from build123d import *

# Parameters (mm, degrees)
SKETCH1_R              = 4.05
BOSS_EXTRUDE1_DEPTH    = 8
SKETCH2_R              = 10
BOSS_EXTRUDE2_DEPTH    = 10
FILLET1_R              = 1
SKETCH3_R              = 2.55
CUT_EXTRUDE1_DEPTH     = 10
CUT_EXTRUDE2_REACH     = 24.891
M2_5_CLEARANCE_HOLE1_D = 2.9
SKETCH28_R             = 3.5
CUT_EXTRUDE3_DEPTH     = 6.5
SKETCH29_W             = 8.1
SKETCH29_H             = 0.5
CUT_EXTRUDE7_DEPTH     = 23.891046451
FILLET2_R              = 0.25
BOSS_EXTRUDE3_START    = 5
BOSS_EXTRUDE3_DEPTH    = 5
CHAMFER1_SIZE          = 0.5
CUT_EXTRUDE8_DEPTH     = 7
BOSS_EXTRUDE4_START    = -2
BOSS_EXTRUDE4_DEPTH    = 3
CHAMFER2_SIZE          = 0.5
SKETCH35_R             = 4.05
CUT_EXTRUDE9_DEPTH     = 8


with BuildPart() as part:
    # Sketch1 → Boss-Extrude1 (new body)
    with BuildSketch(Plane(origin=(0, 0, 0), x_dir=(1, 0, 0), z_dir=(0, 1, 0))):
        with Locations(Location((0, 0, 0), (0, 0, 270))):
            Circle(SKETCH1_R)
    extrude(amount=BOSS_EXTRUDE1_DEPTH)

    # Sketch2 → Boss-Extrude2 (add)
    with BuildSketch(Plane(origin=(0, 8, 0), x_dir=(1, 0, 0), z_dir=(0, 1, 0))):
        with Locations(Location((0, 0, 0), (0, 0, 270))):
            Circle(SKETCH2_R)
    extrude(amount=BOSS_EXTRUDE2_DEPTH)

    # Fillet1
    fillet1_edges = [part.edges().sort_by_distance(p)[0] for p in [
        (0, 0, -4.05),
        (0, 8, -10),
        (0, 18, -10),
    ]]
    fillet(fillet1_edges, radius=FILLET1_R)

    # Sketch3 → Cut-Extrude1 (cut)
    with BuildSketch(Plane(origin=(0, 18, 0), x_dir=(1, 0, 0), z_dir=(0, 1, 0))):
        with Locations(Location((0, 0, 0), (0, 0, 270))):
            Circle(SKETCH3_R)
    extrude(amount=-CUT_EXTRUDE1_DEPTH, mode=Mode.SUBTRACT)

    # Cut-Extrude2: up to this face of the body (flat: up to its plane)
    cut_extrude2_end = Plane(part.part.faces().sort_by_distance((0, 8, -8.745441559))[0])
    # Sketch20 → Cut-Extrude2 (cut, up to the picked face)
    with BuildSketch(Plane(origin=(0, 18, 0), x_dir=(1, 0, 0), z_dir=(0, 1, 0)), mode=Mode.PRIVATE) as cut_extrude2_sk1:
        with BuildLine():
            Line((-0.75, 2.437211521), (0.75, 2.437211521))
            Line((0.75, 2.437211521), (0.75, 9.971835338))
            ThreePointArc((0.75, 9.971835338), (0, 10), (-0.75, 9.971835338))
            Line((-0.75, 9.971835338), (-0.75, 2.437211521))
        make_face()
    cut_extrude2_tool1 = split(extrude(cut_extrude2_sk1.sketch, amount=-CUT_EXTRUDE2_REACH, mode=Mode.PRIVATE), bisect_by=cut_extrude2_end, keep=Keep.BOTH, mode=Mode.PRIVATE)
    add(cut_extrude2_tool1.solids().sort_by(Axis((0, 18, -6.213919), (0, -1, 0)))[0], mode=Mode.SUBTRACT)

    # M2.5 Clearance Hole1 (through all)
    with Locations(Plane(origin=(10, 0, 0), x_dir=(0, 0, -1), z_dir=(1, 0, 0))):
        with Locations((6.204523429, 13)):
            Hole(M2_5_CLEARANCE_HOLE1_D / 2)

    # Sketch28 → Cut-Extrude3 (cut)
    with BuildSketch(Plane(origin=(10, 0, 0), x_dir=(0, 0, -1), z_dir=(1, 0, 0))):
        with Locations((6.204523429, 13)):
            Circle(SKETCH28_R)
    extrude(amount=-CUT_EXTRUDE3_DEPTH, mode=Mode.SUBTRACT)

    # Sketch29 → Cut-Extrude7 (cut, through all)
    with BuildSketch(Plane.XY):
        with Locations((0, 7.75)):
            Rectangle(SKETCH29_W, SKETCH29_H)
    extrude(amount=-CUT_EXTRUDE7_DEPTH, mode=Mode.SUBTRACT)

    # Fillet2
    fillet2_edges = [part.edges().sort_by_distance(p)[0] for p in [
        (-3.3, 8, 0),
        (3.3, 8, 0),
        (0, 7.5, 0),
    ]]
    fillet(fillet2_edges, radius=FILLET2_R - 0.0001)  # a hair under: the kernel refuses the full size

    # Sketch30 → Boss-Extrude3 (add)
    with BuildSketch(Plane(origin=(0, 18, 0), x_dir=(1, 0, 0), z_dir=(0, 1, 0)).offset(BOSS_EXTRUDE3_START)):
        with BuildLine():
            Line((-0.75, 3.31624788), (-0.75, 2.437211521))
            ThreePointArc((-0.75, 2.437211521), (0, -2.55), (0.75, 2.437211521))
            Line((0.75, 2.437211521), (0.75, 3.31624788))
            ThreePointArc((0.75, 3.31624788), (0, -3.4), (-0.75, 3.31624788))
        make_face()
    extrude(amount=-BOSS_EXTRUDE3_DEPTH)

    # Chamfer1
    chamfer1_edges = [part.edges().sort_by_distance(p)[0] for p in [
        (0, 23, 3.4),
    ]]
    chamfer(chamfer1_edges, length=CHAMFER1_SIZE)

    # Sketch33 → Cut-Extrude8 (cut)
    with BuildSketch(Plane.ZY.offset(10)):
        Polygon((-3.144567003, 13), (-4.674545216, 15.65), (-7.734501643, 15.65), (-9.264479856, 13), (-7.734501643, 10.35), (-4.674545216, 10.35), align=None)
    extrude(amount=-CUT_EXTRUDE8_DEPTH, mode=Mode.SUBTRACT)

    # Sketch34 → Boss-Extrude4 (add)
    with BuildSketch(Plane(origin=(0, 23, 0), x_dir=(1, 0, 0), z_dir=(0, 1, 0)).offset(BOSS_EXTRUDE4_START)):
        with BuildLine():
            Line((-0.75, 3.31624788), (-0.75, 4.132493194))
            ThreePointArc((-0.75, 4.132493194), (0, -4.2), (0.75, 4.132493194))
            Line((0.75, 4.132493194), (0.75, 3.31624788))
            ThreePointArc((0.75, 3.31624788), (0, -3.4), (-0.75, 3.31624788))
        make_face()
    extrude(amount=-BOSS_EXTRUDE4_DEPTH)

    # Chamfer2
    chamfer2_edges = [part.edges().sort_by_distance(p)[0] for p in [
        (0, 21, 4.2),
    ]]
    chamfer(chamfer2_edges, length=CHAMFER2_SIZE)

    # Sketch35 → Cut-Extrude9 (cut)
    with BuildSketch(Plane.XZ):
        Circle(SKETCH35_R)
    extrude(amount=-CUT_EXTRUDE9_DEPTH, mode=Mode.SUBTRACT)


solid = part.part
Here's how the part is built. I have some questions about the finished solid (model axes, mm). A direction names the side the tool comes from. Give positions to 0.01 mm unless a question says otherwise; leave off trailing zeros. Order: outer loops, then holes, each group sorted by start corner. A loop starts at its lowest first (then second) coordinate and runs counter-clockwise, first axis right, second up. Notation, with made-up numbers: (34, -1.75) -> (52, -1.75) arc R28 cw to (52, 32.25) -> close; hole circle Ø10 at (80.5, 4.5). An arc over 180 degrees is marked (long way). Use a Markdown table: item, result. Add a question column.
Item 1: Will these pins go through, and if not, where does the flat tip stop? pin 1 (2 mm diameter, centred on y = 13, z = -5.5, fed in from +X); pin 2 (6 mm diameter, centred on y = 12, z = -5.5, fed in from +X); pin 3 (3 mm diameter, centred on x = 6, y = 13, fed in from +Z).
Item 2: Imagine slicing it at B-B on y = 12.5. Please give me the cut outline in (x, z), plus the area to 3 significant figures.
Item 3: Imagine slicing it at C-C on x = 1.25. Give the number of separate pieces and of enclosed holes in the cut face, plus the area to 3 significant figures.
Item 4: If we mould it in two halves opening along Z, with no side actions, what happens to faces 6 (the face through (-2, 8, 2)), 7 (the face through (0.1, 21.8, 3.4)), 8 (the face through (-3, 14.2, -4.9))? For each: pulls with the +Z half, pulls with the -Z half, needs draft (parallel to the pull), parting line crosses it, or undercut.
Item 5: I need wall thicknesses on line 1 (X direction, y = 11, z = 0); line 2 (X direction, y = 19.45, z = 0); line 3 (Y direction, x = 3, z = -4). Which ranges of each line are inside material? Lowest first, please.
Item 6: Imagine slicing it at D-D on y = 19.5. Please give me the cut outline in (x, z), plus the area to 3 significant figures.
Item 7: For faces 1 (the face through (-6.29, 14.31, -3.9)), 2 (the face through (-1.891, 12.118, -7.355)), 3 (the face through (0.75, 13.9, -4.6)), 4 (the face through (3.5, 15, -6)), 5 (the face through (-2, 18, 4)), which set-ups out of +Z, -Z, +X, -X, +Y, -Y let a thin tool reach every point of the face, with its end or its side?
Item 8: Imagine slicing it at A-A on z = 0. Please give me the cut outline in (x, y), plus the area to 3 significant figures.
Data:
| question | item | result |
|---|---|---|
| 1 | pin 1 | stops at x = 3.5 |
| 1 | pin 2 | stops at x = 9.68 |
| 1 | pin 3 | stops at z = 8.93 |
| 2 | outline | (-9.39, -3.43) -> (-3, -3.43) -> (-3, -4.84) -> (-0.75, -4.84) -> (-0.75, -2.44) arc R2.55 cw (long way) to (0.75, -2.44) -> (0.75, -4.84) -> (3.5, -4.84) -> (3.5, -2.74) -> (9.62, -2.74) arc R10 ccw (long way) to start; (-4.41, -8.98) arc R10 ccw to (-0.75, -9.97) -> (-0.75, -7.57) -> (-3, -7.57) -> (-3, -8.98) -> close; (0.75, -9.97) arc R10 ccw to (3.5, -9.37) -> (3.5, -7.57) -> (0.75, -7.57) -> close |
| 2 | area | 217 mm² |
| 3 | separate pieces | 2 |
| 3 | enclosed holes | 1 |
| 3 | area | 160 mm² |
| 4 | face 6 | needs draft |
| 4 | face 7 | parting line crosses it |
| 4 | face 8 | undercut |
| 5 | line 1 | x = -10 to -2.55, 2.55 to 10 |
| 5 | line 2 | x = -4.2 to -2.55, 2.55 to 4.2 |
| 5 | line 3 | y = 8 to 18 |
| 6 | outline | (-0.75, -4.13) -> (-0.75, -2.44) arc R2.55 cw (long way) to (0.75, -2.44) -> (0.75, -4.13) arc R4.2 ccw (long way) to start |
| 6 | area | 32.5 mm² |
| 7 | face 1 | -X |
| 7 | face 2 | +X, -X |
| 7 | face 3 | -Z, +Y, -Y |
| 7 | face 4 | +X |
| 7 | face 5 | +Y |
| 8 | outline | (-10, 9) arc R1 ccw to (-9, 8) -> (-2.55, 8) -> (-2.55, 23) -> (-2.9, 23) -> (-3.4, 22.5) -> (-3.4, 21) -> (-3.7, 21) -> (-4.2, 20.5) -> (-4.2, 18) -> (-9, 18) arc R1 ccw to (-10, 17) -> close; (2.55, 8) -> (9, 8) arc R1 ccw to (10, 9) -> (10, 17) arc R1 ccw to (9, 18) -> (4.2, 18) -> (4.2, 20.5) -> (3.7, 21) -> (3.4, 21) -> (3.4, 22.5) -> (2.9, 23) -> (2.55, 23) -> close |
| 8 | area | 161 mm² |
